```python
from build123d import *

# Parameters (mm, degrees)
BOSS_EXTRUDE1_DEPTH       = 55
BOSS_EXTRUDE2_DEPTH       = 5
F_4_0MM_DOWEL_HOLE1_D     = 4
F_4_0MM_DOWEL_HOLE1_DEPTH = 20
F_4_0MM_DOWEL_HOLE1_TIP   = 1.201721238
FILLET3_R                 = 1
FILLET4_R                 = 1
FILLET5_R                 = 0.5
FILLET6_R                 = 0.5


with BuildPart() as part:
    # Sketch1 → Boss-Extrude1 (new body)
    with BuildSketch(Plane(origin=(0, 0, 0), x_dir=(1, 0, 0), z_dir=(0, 1, 0))):
        Polygon((3.897114317, -6.75), (7.794228634, 0), (3.897114317, 6.75), (-3.897114317, 6.75), (-7.794228634, 0), (-3.897114317, -6.75), align=None)
    extrude(amount=BOSS_EXTRUDE1_DEPTH)

    # Sketch2 → Boss-Extrude2 (add)
    with BuildSketch(Plane.XZ):
        Polygon((5.051814855, -8.75), (10.103629711, 0), (5.051814855, 8.75), (-5.051814855, 8.75), (-10.103629711, 0), (-5.051814855, -8.75), align=None)
    extrude(amount=BOSS_EXTRUDE2_DEPTH)

    # Ø4.0mm Dowel Hole1
    with Locations(Plane(origin=(0, 55, 0), x_dir=(1, 0, 0), z_dir=(0, 1, 0))):
        with Locations((0, 0)):
            Hole(F_4_0MM_DOWEL_HOLE1_D / 2, depth=F_4_0MM_DOWEL_HOLE1_DEPTH)
            with Locations((0, 0, -(F_4_0MM_DOWEL_HOLE1_DEPTH + F_4_0MM_DOWEL_HOLE1_TIP / 2))):  # 118° drill point
                Cone(0, F_4_0MM_DOWEL_HOLE1_D / 2, F_4_0MM_DOWEL_HOLE1_TIP, mode=Mode.SUBTRACT)

    # Fillet3
    fillet3_edges = [part.edges().sort_by_distance(p)[0] for p in [
        (-3.897114317, 27.5, 6.75),
        (-7.794228634, 27.5, 0),
        (-3.897114317, 27.5, -6.75),
        (3.897114317, 27.5, -6.75),
        (7.794228634, 27.5, 0),
        (3.897114317, 27.5, 6.75),
    ]]
    fillet(fillet3_edges, radius=FILLET3_R)

    # Fillet4
    fillet4_edges = [part.edges().sort_by_distance(p)[0] for p in [
        (-5.051814855, -2.5, -8.75),
        (5.051814855, -2.5, -8.75),
        (10.103629711, -2.5, 0),
        (5.051814855, -2.5, 8.75),
        (-5.051814855, -2.5, 8.75),
        (-10.103629711, -2.5, 0),
    ]]
    fillet(fillet4_edges, radius=FILLET4_R)

    # Fillet5
    fillet5_edges = [part.edges().sort_by_distance(p)[0] for p in [
        (4.974464586, -5, 8.616025404),
        (9.948929172, -5, 0),
        (4.974464586, -5, -8.616025404),
        (-5.845671476, 0, -3.375),
        (0, 0, -6.75),
        (5.845671476, 0, -3.375),
        (5.845671476, 0, 3.375),
        (0, 0, 6.75),
        (-5.845671476, 0, 3.375),
        (-3.819764048, 0, -6.616025404),
        (3.819764048, 0, -6.616025404),
        (7.639528096, 0, 0),
        (3.819764048, 0, 6.616025404),
        (-3.819764048, 0, 6.616025404),
        (-7.639528096, 0, 0),
        (7.577722283, 0, -4.375),
        (7.577722283, -5, -4.375),
        (0, 0, -8.75),
        (-7.577722283, 0, -4.375),
        (-7.577722283, 0, 4.375),
        (0, 0, 8.75),
        (7.577722283, 0, 4.375),
        (-4.974464586, 0, -8.616025404),
        (-9.948929172, 0, 0),
        (-4.974464586, 0, 8.616025404),
        (4.974464586, 0, 8.616025404),
        (9.948929172, 0, 0),
        (4.974464586, 0, -8.616025404),
        (0, -5, -8.75),
        (7.577722283, -5, 4.375),
        (0, -5, 8.75),
        (-7.577722283, -5, 4.375),
        (-7.577722283, -5, -4.375),
        (-4.974464586, -5, -8.616025404),
        (-9.948929172, -5, 0),
        (-4.974464586, -5, 8.616025404),
    ]]
    fillet(fillet5_edges, radius=FILLET5_R)

    # Fillet6
    fillet6_edges = [part.edges().sort_by_distance(p)[0] for p in [
        (-5.845671476, 55, -3.375),
        (0, 55, -6.75),
        (0, 55, 6.75),
        (5.845671476, 55, 3.375),
        (5.845671476, 55, -3.375),
        (-5.845671476, 55, 3.375),
        (-7.639528096, 55, 0),
        (-3.819764048, 55, 6.616025404),
        (3.819764048, 55, 6.616025404),
        (7.639528096, 55, 0),
        (3.819764048, 55, -6.616025404),
        (-3.819764048, 55, -6.616025404),
    ]]
    fillet(fillet6_edges, radius=FILLET6_R)


solid = part.part
```
Model file for the job. Use its own axes, mm. A direction names the side the tool comes from. Give positions to 0.01 mm unless a question says otherwise; leave off trailing zeros. Loops run counter-clockwise (first coordinate to the right, second up) from the corner with the lowest first, then second, coordinate; pieces in that order, holes last. Notation, with made-up numbers: M 16.25,-13.75 L 31.25,-13.75 A9 cw 31.25,-5.75 Z; hole C 58.5,-24 d8. An arc over 180 degrees is marked long. Use one line per item in the form item = value.
Item 1: Which spindle directions (+Z, -Z, +X, -X, +Y, -Y) get a long thin tool onto all of the face, cutting with end or side? Do faces 1 (the cylindrical face through (-7.64, 27.88, 0.01)), 2 (the cylindrical face through (5.7, 54.85, -3.34)), 3 (the flat face through (-5.87, 27.12, 3.33)), 4 (the flat face through (0, 27, 6.75)), 5 (the flat face through (5.82, 27.12, 3.42)). Say none if no direction does.
Filled in:
face_1 = -X, +Y
face_2 = -Z, +X, +Y
face_3 = +Z, -X, +Y
face_4 = +Z, +X, -X, +Y
face_5 = +Z, +X, +Y
Item 2: Drill centre lines: L1, parallel to Z at x = 0, y = 51.25; L2, parallel to Y at x = 4.75, z = 7; L3, parallel to Y at x = -4, z = 5.75. Where is each one in solid material? Low to high.
Filled in:
L1 = -6.75 to -2, 2 to 6.75
L2 = -5 to 0
L3 = -5 to 54.99
Item 3: Slice it at B-B on y = 27. List the corners of the cut face in (x, z).
Filled in:
outline = M -7.51,-0.5 L -4.19,-6.25 A1 ccw -3.32,-6.75 L 3.32,-6.75 A1 ccw 4.19,-6.25 L 7.51,-0.5 A1 ccw 7.51,0.5 L 4.19,6.25 A1 ccw 3.32,6.75 L -3.32,6.75 A1 ccw -4.19,6.25 L -7.51,0.5 A1 ccw Z
Item 4: Slice it at A-A on y = 51. List the corners of the cut face in (x, z).
Filled in:
outline = M -7.51,-0.5 L -4.19,-6.25 A1 ccw -3.32,-6.75 L 3.32,-6.75 A1 ccw 4.19,-6.25 L 7.51,-0.5 A1 ccw 7.51,0.5 L 4.19,6.25 A1 ccw 3.32,6.75 L -3.32,6.75 A1 ccw -4.19,6.25 L -7.51,0.5 A1 ccw Z; hole C 0,0 d4
Item 5: Flat gauge pins, fed straight in: pin 1 Ø10 at (y, z) = (37.5, -5.5) entering from -X; pin 2 Ø2 at (x, y) = (-4.5, 21.5) entering from -Z; pin 3 Ø7.5 at (x, y) = (0, 24) entering from +Z. Where does each tip first touch, or does it go through?
Filled in:
pin_1 = -7.51
pin_2 = -6.73
pin_3 = 6.75
